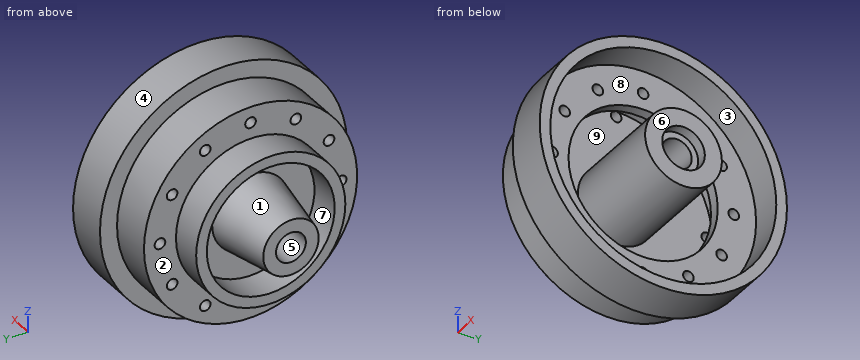
from build123d import *

# Parameters (mm, degrees)
SCHIZZO2_R                  = 2.5
TAGLIO_ESTRUSIONE1_DEPTH    = 56
RIPETIZIONECIRCOLARE1_COUNT = 12


with BuildPart() as part:
    # Schizzo1 → Rivoluzione1 (revolve)
    with BuildSketch(Plane.XY):
        Polygon((-35, 7), (45, 7), (45, 10), (50, 10), (50, 18), (0.0029942, 18), (0.0029942, 45), (15, 45), (15, 35), (20, 35), (20, 53), (35, 53), (35, 58), (15, 58), (15, 50), (-5, 50), (-5, 35), (-20, 35), (-20, 30), (-5, 30), (-5, 18), (-35, 13), align=None)
    revolve(axis=Axis((-44.939802223, 0, 0), (1, 0, 0)))

    # Schizzo2 → Taglio-Estrusione1 (cut, through all)
    with BuildSketch(Plane.ZY.offset(5)):
        with Locations((0, -42.5)):
            Circle(SCHIZZO2_R)
    taglio_estrusione1 = extrude(amount=-TAGLIO_ESTRUSIONE1_DEPTH, mode=Mode.SUBTRACT)

    # RipetizioneCircolare1: Taglio-Estrusione1 ×12 about axis
    ripetizionecircolare1_axis = Axis((0, 0, 0), (1, 0, 0))
    for i in range(1, RIPETIZIONECIRCOLARE1_COUNT):
        add(taglio_estrusione1.rotate(ripetizionecircolare1_axis, i * 360 / RIPETIZIONECIRCOLARE1_COUNT), mode=Mode.SUBTRACT)


solid = part.part
Source: CAD feature listing. Evaluate the final solid. Frame: model axes, mm. Face numbers are marked on the shaded views. A direction names the side the tool comes from. Coordinates: 2 decimals unless noted, no trailing zeros. Order: outer loops, then holes, each group sorted by start corner. A loop starts at its lowest first (then second) coordinate and runs counter-clockwise, first axis right, second up. Notation, with made-up numbers: M 14.25,62 L 22.25,62 A34 ccw 22.25,99 Z; hole C -34,-37.5 d9. An arc over 180 degrees is marked long. Write each question's results on one line, items separated by ' | '. Start each with the question number.
Item 1: Cut plane A-A (y = 42.5). Return loops of the section in (x, z), and give its area (3 significant figures).
Item 2: Draft query along Y for the marked faces 1, 2, 3 and 4. Return one class per face: pulls with the +Y half, pulls with the -Y half, needs draft (parallel to the pull), parting line crosses it, or undercut.
Item 3: Cut plane B-B (x = 28.5). Return loops of the section in (y, z).
Item 4: Cut plane C-C (y = -27.5). Return loops of the section in (x, z).
Item 5: Cut plane D-D (x = -3.5). Count the separate pieces of the cut face and the enclosed holes in it, and give its area (3 significant figures).
Item 6: First-contact query: pin 1 Ø3 at (y, z) = (12, -42) entering from -X; pin 2 Ø5 at (x, y) = (12, -29.5) entering from +Z; pin 3 Ø1 at (x, z) = (11.5, 41.5) entering from -Y. Flat tips, straight axial feed; report the tip coordinate or a pass-through.
Item 7: Line query: probe 1 along X at (y, z) = (42, -16); probe 2 along Y at (x, z) = (33, -16.5); probe 3 along Y at (x, z) = (-1.9, -21.25). Output: solid intervals per line, ascending.
Item 8: Set-up query: the marked faces 5, 6, 7, 8 and 9. Return all of +Z, -Z, +X, -X, +Y, -Y with unobstructed straight access to the full face (end or side cutting, diameter ignored); none if empty.
Checked values:
1) outline: M -5,-26.34 L 15,-26.34 L 15,-39.47 L 35,-39.47 L 35,-31.67 L 20,-31.67 L 20,-2.5 L 15,-2.5 L 15,-14.79 L 0,-14.79 L 0,-2.5 L -5,-2.5 Z; M -5,2.5 L 0,2.5 L 0,14.79 L 15,14.79 L 15,2.5 L 20,2.5 L 20,31.67 L 35,31.67 L 35,39.47 L 15,39.47 L 15,26.34 L -5,26.34 Z | area: 1,190 mm2
2) face 1: undercut | face 2: needs draft | face 3: undercut | face 4: parting line crosses it
3) outline: C 0,0 d116; C 0,0 d36; hole C 0,0 d106; hole C 0,0 d14
4) outline: M -20,-21.65 L -5,-21.65 L -5,-41.76 L 15,-41.76 L 15,-51.07 L 35,-51.07 L 35,-45.31 L 20,-45.31 L 20,-21.65 L 15,-21.65 L 15,-35.62 L 0,-35.62 L 0,35.62 L 15,35.62 L 15,21.65 L 20,21.65 L 20,45.31 L 35,45.31 L 35,51.07 L 15,51.07 L 15,41.76 L -5,41.76 L -5,21.65 L -20,21.65 L -20,11.99 L -5,11.99 L -5,-11.99 L -20,-11.99 Z
5) separate pieces: 1 | enclosed holes: 13 | area: 7,460 mm2
6) pin 1: stops at x = -5 | pin 2: stops at z = 42.08 | pin 3: stops at y = -28.62
7) probe 1: x = -5 to 0, 15 to 20 | probe 2: y = -55.6 to -50.37, -7.19 to 7.19, 50.37 to 55.6 | probe 3: y = -45.26 to -39.31, -34.31 to 34.31, 39.31 to 45.26
8) face 5: +X, -X | face 6: +Z, -Z, +X, +Y, -Y | face 7: -X | face 8: +X | face 9: none
